Source: three-view drawing plus pictorial views. Frame: mm from the lowest corner of the part. Coordinates: 2 decimals unless noted, no trailing zeros. Order: outer loops, then holes, each group sorted by start corner. A loop starts at its lowest first (then second) coordinate and runs counter-clockwise, first axis right, second up. Notation, with made-up numbers: (25, 86.25) -> (32, 86.25) arc R22 ccw to (32, 110.25) -> close; hole circle Ø1 at (-29, 11). An arc over 180 degrees is marked (long way). Use CSV: the item, a comma, the result in double quotes. Start each with the question number.
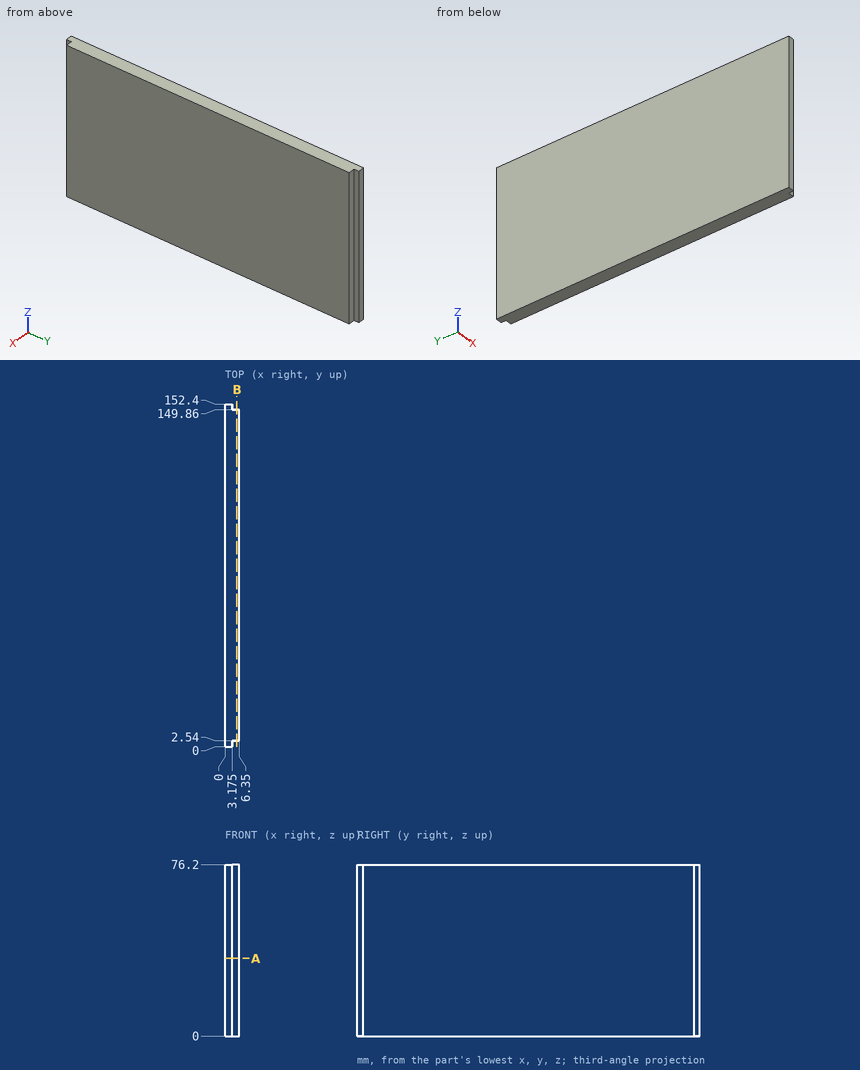
1. Section A-A on z = 34.5. Return loops of the section in (x, y) (3 decimals).
2. Contact query for flat-ended pins moving along their axis: P1, Ø1.6, axis at x = 4.5, z = 45.5, coming from the -Y side; P2, Ø0.8, axis at y = 1, z = 21.5, coming from the +X side (3 decimals); P3, Ø1.5, axis at x = 5, z = 25, coming from the +Y side. Output: stop coordinate, or through.
3. Section B-B on x = 5.25. Return loops of the section in (y, z), then the cut area to 3 significant figures.
4. Material intervals for line 1 along Y through (x, z) = (4, 21.5), sorted ascending.
Values follow:
1,outline,"(0, 0) -> (3.175, 0) -> (3.175, 2.54) -> (6.35, 2.54) -> (6.35, 149.86) -> (3.175, 149.86) -> (3.175, 152.4) -> (0, 152.4) -> close"
2,P1,"stops at y = 2.54"
2,P2,"stops at x = 3.175"
2,P3,"stops at y = 149.86"
3,outline,"(2.54, 0) -> (149.86, 0) -> (149.86, 76.2) -> (2.54, 76.2) -> close"
3,area,"11,200 mm2"
4,line 1,"y = 2.54 to 149.86"
